```python
from build123d import *

# Parameters (mm, degrees)
ESQUISSE1_W        = 380
ESQUISSE1_H        = 380
ESQUISSE1_W_2      = 340
ESQUISSE1_H_2      = 340
BOSS_EXTRU_1_DEPTH = 210
ESQUISSE2_W        = 380
ESQUISSE2_H        = 380
BOSS_EXTRU_2_DEPTH = 20


with BuildPart() as part:
    # Esquisse1 → Boss.-Extru.1 (new body)
    with BuildSketch(Plane.XY):
        Rectangle(ESQUISSE1_W, ESQUISSE1_H)
        Rectangle(ESQUISSE1_W_2, ESQUISSE1_H_2, mode=Mode.SUBTRACT)
    extrude(amount=BOSS_EXTRU_1_DEPTH)

    # Esquisse2 → Boss.-Extru.2 (add)
    with BuildSketch(Plane.XY.offset(210)):
        Rectangle(ESQUISSE2_W, ESQUISSE2_H)
    extrude(amount=BOSS_EXTRU_2_DEPTH)


solid = part.part
```
CAD build for the part. Positions are in the model's coordinates, mm. A direction names the side the tool comes from. Coordinates: 2 decimals unless noted, no trailing zeros. Write each loop counter-clockwise with the first axis right and the second up, starting at its lowest first coordinate (ties: lowest second). Pieces come first, ordered by that corner, then holes. Notation, with made-up numbers: (37.25, 60.5) -> (54.25, 60.5) arc R6 cw to (54.25, 66.5) -> close; hole circle Ø4 at (49, -16.75). An arc over 180 degrees is marked (long way). Return JSON: item names as keys, results as strings. Group by question number.
Q1. Flat gauge pin, fed straight in: pin 1 (1 mm diameter, centred on x = -139, y = 132.5, fed in from -Z). Where does the tip first touch, or does it go through?
Q2. Cut at C-C, the plane z = 79.5. Give the cut face in (x, y).
Q3. Pull direction X, two halves, no side cores. Call faces 3 (the face through (-2, -170, 104)), 4 (the face through (-3, 3, 230)), 5 (the face through (-190, -3, 113)): released by +X, released by -X, zero draft, split by the parting line, or undercut.
Q4. Cut at A-A, the plane y = -125. Give the cut face in (x, z).
Q5. Drill centre lines: line 1 (X direction, y = 26.5, z = 89); line 2 (Z direction, x = 73, y = 16.5). Where is each one in solid material? Low to high.
Q6. Which spindle directions (+Z, -Z, +X, -X, +Y, -Y) get a long thin tool onto all of the face, cutting with end or side? Do faces 1 (the face through (170, -2, 104)), 2 (the face through (-3, -190, 113)). Say none if no direction does.
Returned:
{
 "1": {"pin 1": "stops at z = 210"},
 "2": {"outline": "(-190, -190) -> (190, -190) -> (190, 190) -> (-190, 190) -> close; hole (-170, -170) -> (170, -170) -> (170, 170) -> (-170, 170) -> close"},
 "3": {"face 3": "undercut", "face 4": "zero draft", "face 5": "released by -X"},
 "4": {"outline": "(-190, 0) -> (-170, 0) -> (-170, 210) -> (170, 210) -> (170, 0) -> (190, 0) -> (190, 230) -> (-190, 230) -> close"},
 "5": {"line 1": "x = -190 to -170, 170 to 190", "line 2": "z = 210 to 230"},
 "6": {"face 1": "-Z", "face 2": "+Z, -Z, +X, -X, -Y"}
}
